Can you work these out from the model? Positions are in its coordinate system, mm. A direction names the side the tool comes from. Give positions to 0.01 mm unless a question says otherwise; leave off trailing zeros. Order: outer loops, then holes, each group sorted by start corner. A loop starts at its lowest first (then second) coordinate and runs counter-clockwise, first axis right, second up. Notation, with made-up numbers: M 41,27.5 L 74,27.5 A22 ccw 74,50.5 Z; hole C 44,43 d10. An arc over 180 degrees is marked long. Use a Markdown table: item, result. Add a question column.
from build123d import *

# Parameters (mm, degrees)
F3_DEPTH = 12.7


# Not quite as in the source:
# - the program builds the solid bodies; features that only make, move or delete a surface that nothing else refers to are left out


with BuildPart() as f3:
    # F2 (on Front) → F3 (new body, symmetric)
    with BuildSketch(Plane.XZ):
        with BuildLine():
            Line((-22.225, 25.4), (-28.3980633142, 25.4))
            ThreePointArc((-28.3980633142, 25.4), (-28.6260297603, 25.1428005632), (-28.8516668522, 24.8835552092))
            Line((-28.8516668522, 24.8835552092), (-38.1, 7.62))
            Line((-38.1, 7.62), (-38.1, 0))
            Line((-38.1, 0), (0, 0))
            Line((0, 0), (0, 7.62))
            Line((0, 7.62), (-22.225, 7.62))
            Line((-22.225, 7.62), (-22.225, 25.4))
        make_face()
        with BuildLine():
            ThreePointArc((-28.8516668522, 24.8835552092), (-28.6260297603, 25.1428005632), (-28.3980633142, 25.4))
            Line((-28.3980633142, 25.4), (-28.575, 25.4))
            Line((-28.575, 25.4), (-28.8516668522, 24.8835552092))
        make_face()
    extrude(amount=F3_DEPTH, both=True)


solid = f3.part
1. If we section it at B-B, the plane x = -21.5: List the corners of the cut face in (y, z) for me, then the cut area to 3 significant figures.
2. If we section it at C-C, the plane z = 22.25: List the corners of the cut face in (x, y) for me (1 decimal), then the cut area to 3 significant figures.
3. I need wall thicknesses on L1, parallel to Z at x = -11, y = -10.75; L2, parallel to Z at x = -32, y = 9; L3, parallel to X at y = 11.25, z = 16.75 (3 decimals). Which ranges of each line are inside material? Lowest first, please. Write a range as [from, to].
4. Will these pins go through, and if not, where does the flat tip stop? pin 1 (5.5 mm diameter, centred on y = -2.5, z = 15.5, fed in from +X) (3 decimals); pin 2 (5 mm diameter, centred on x = -10.5, y = 9.5, fed in from +Z).
5. On a 3-axis mill with a long thin cutter (end or side, diameter ignored), from which of +Z, -Z, +X, -X, +Y, -Y can I reach the whole of each face in a straight line? I mean faces 1 (the face through (-24, -12.7, 10)), 2 (the face through (-22.225, 0, 16)). Say none if no direction works.
6. If we section it at A-A, the plane y = -9.5: List the corners of the cut face in (x, z) for me (3 decimals), then the cut area to 3 significant figures.
Geometry results:
| question | item | result |
|---|---|---|
| 1 | outline | M -12.7,0 L 12.7,0 L 12.7,7.62 L -12.7,7.62 Z |
| 1 | area | 194 mm^2 |
| 2 | outline | M -30.3,-12.7 L -22.2,-12.7 L -22.2,12.7 L -30.3,12.7 Z |
| 2 | area | 204 mm^2 |
| 3 | L1 | z = [0, 7.62] |
| 3 | L2 | z = [0, 19.01] |
| 3 | L3 | x = [-33.209, -22.225] |
| 4 | pin 1 | stops at x = -22.225 |
| 4 | pin 2 | stops at z = 7.62 |
| 5 | face 1 | +Z, -Z, +X, -X, -Y |
| 5 | face 2 | +Z, +X, +Y, -Y |
| 6 | outline | M -38.1,0 L 0,0 L 0,7.62 L -22.225,7.62 L -22.225,25.4 L -28.575,25.4 L -38.1,7.62 Z |
| 6 | area | 488 mm^2 |
